Model file for the job. Use its own axes, mm. A direction names the side the tool comes from. Round coordinates to 2 decimals unless told otherwise and drop trailing zeros. Loops run counter-clockwise (first coordinate to the right, second up) from the corner with the lowest first, then second, coordinate; pieces in that order, holes last. Notation, with made-up numbers: M -19,61 L 24,61 A26 cw 24,98 Z; hole C 39.25,55 d6. An arc over 180 degrees is marked long. Use a Markdown table: item, result. Add a question column.
Item 1: Saw through at C-C on y = -239. Write the cut outline in (x, z).
Item 2: Tool access for faces 1 (the flat face through (-122, -197, 14.158)), 2 (the flat face through (-100, -220, -75.842)), 3 (the flat face through (-151.12, -291.64, 66.76)): list every direction of +Z, -Z, +X, -X, +Y, -Y with a clear straight run to the whole face (end or side of a thin tool).
Item 3: Saw through at B-B on x = -86.5. Write the cut outline in (y, z).
Item 4: Pin check, flat tips, straight feed: P1, Ø9.5, axis at x = 13, y = -14.5, coming from the +Z side; P2, Ø15.5, axis at x = -306, y = -333.5, coming from the -Z side; P3, Ø10, axis at x = -260.5, z = 41.5, coming from the -Y side; P4, Ø10, axis at y = -299.5, z = -12.5, coming from the +X side. Stop position of each tip, or through.
Item 5: Wall check: L1, parallel to Z at x = -208, y = -295; L2, parallel to Z at x = -193.5, y = -272; L3, parallel to X at y = -329, z = -60. Give the ranges that are in metal, low to high. Write a range as from..to.
Item 6: Two-plate mould, pull along Y, no slides. Class faces 4 (the flat face through (-27.86, -168.38, 66.76)), 5 (the cylindrical face through (34.67, -15.25, -43.1)), 6 (the flat face through (-304, -337, 59.158)), 7 (the flat face through (-264.9, -309.65, 0)): +Y half, -Y half, draft (parallel to the pull), parting line (faces both ways), or undercut.
Item 7: Saw through at D-D on z = 29. Write the cut outline in (x, y).
Item 8: Saw through at A-A on z = 6.5. Write the cut outline in (x, y), then the cut area to 3 significant figures.
```python
from build123d import *

# Parameters (mm, degrees)
F1_ANGLE       = 90
F2_W           = 35
F2_H           = 35
F2_R           = 7.5
F3_ANGLE       = 5
F4_ANGLE_START = 270
F4_ANGLE       = 5
F5_W           = 10
F5_H           = 120
F6_ANGLE_START = 280
F6_ANGLE       = 70
F7_W           = 35
F7_H           = 15
F8_ANGLE_START = 30
F8_ANGLE       = 30
F10_DEPTH      = 15


with BuildPart() as f1:
    # F0 (on Front) → F1 (revolve)
    with BuildSketch(Plane.XZ):
        Polygon((0, -75.8424619118), (0, 74.1575380882), (-42.5, 74.1575380882), (-42.5, 14.1575380882), (-32.5, 14.1575380882), (-32.5, 59.1575380882), (-10, 59.1575380882), (-10, -75.8424619118), align=None)
    revolve(axis=Axis((-319.5, 0, -5.3764432669), (0, 0, -1)), revolution_arc=F1_ANGLE)

    # F2 (on face) → F3 (revolve)
    with BuildSketch(Plane(origin=(-319.5, 0, 0), x_dir=(0, -1, 0), z_dir=(-1, 0, 0))):
        with Locations((337, 41.6575380882)):
            Rectangle(F2_W, F2_H)
        with Locations((337, 41.6575380882)):
            Circle(F2_R, mode=Mode.SUBTRACT)
        with Locations((337, -43.3424619118)):
            Rectangle(F2_W, F2_H)
        with Locations((337, -43.3424619118)):
            Circle(F2_R, mode=Mode.SUBTRACT)
    revolve(axis=Axis((-319.5, 0, 7.2890669107), (0, 0, 1)), revolution_arc=F3_ANGLE)

    # F2 (on face) → F4 (revolve)
    with BuildSketch(Plane(origin=(-319.5, 0, 0), x_dir=(0, -1, 0), z_dir=(-1, 0, 0)), mode=Mode.PRIVATE) as f4_sk:
        with Locations((337, 41.6575380882)):
            Rectangle(F2_W, F2_H)
        with Locations((337, 41.6575380882)):
            Circle(F2_R, mode=Mode.SUBTRACT)
        with Locations((337, -43.3424619118)):
            Rectangle(F2_W, F2_H)
        with Locations((337, -43.3424619118)):
            Circle(F2_R, mode=Mode.SUBTRACT)
    revolve(f4_sk.sketch.rotate(Axis((-319.5, 0, 74.1575380882), (0, 0, -1)), F4_ANGLE_START), axis=Axis((-319.5, 0, 74.1575380882), (0, 0, -1)), revolution_arc=F4_ANGLE)

    # F5 (on Front) → F6 (revolve, cut)
    with BuildSketch(Plane.XZ, mode=Mode.PRIVATE) as f6_sk:
        with Locations((-5, -0.8424619118)):
            Rectangle(F5_W, F5_H)
    revolve(f6_sk.sketch.rotate(Axis((-319.5, 0, -29.9057289958), (0, 0, 1)), F6_ANGLE_START), axis=Axis((-319.5, 0, -29.9057289958), (0, 0, 1)), revolution_arc=F6_ANGLE, mode=Mode.SUBTRACT)

    # F7 (on Front) → F8 (revolve)
    with BuildSketch(Plane.XZ, mode=Mode.PRIVATE) as f8_sk:
        with Locations((17.5, 66.6575380882)):
            Rectangle(F7_W, F7_H)
    revolve(f8_sk.sketch.rotate(Axis((-319.5, 0, -44.4073081017), (0, 0, -1)), F8_ANGLE_START), axis=Axis((-319.5, 0, -44.4073081017), (0, 0, -1)), revolution_arc=F8_ANGLE)

    # F9 (on face) → F10 (cut)
    with BuildSketch(Plane.XY.offset(74.1575380882)):
        with BuildLine():
            ThreePointArc((-128.7858349133, -272.3680547261), (-123.9019759301, -268.8822474243), (-119.0818139536, -265.3088779176))
            ThreePointArc((-119.0818139536, -265.3088779176), (-126.8087717489, -260.5320409865), (-135.6687521495, -262.5382301946))
            Line((-135.6687521495, -262.5382301946), (-128.7858349133, -272.3680547261))
        make_face()
        with BuildLine():
            ThreePointArc((-138.7382619085, -279.07247095), (-125.2807759939, -283.8447512008), (-116.7858349133, -272.3680547261))
            ThreePointArc((-116.7858349133, -272.3680547261), (-117.3742563302, -268.6564682402), (-119.0818139536, -265.3088779176))
            ThreePointArc((-119.0818139536, -265.3088779176), (-123.9019759301, -268.8822474243), (-128.7858349133, -272.3680547261))
            ThreePointArc((-128.7858349133, -272.3680547261), (-133.7318004616, -275.7651646606), (-138.7382619085, -279.07247095))
        make_face()
        with BuildLine():
            ThreePointArc((-135.6687521495, -262.5382301946), (-140.5842451107, -270.1777312768), (-138.7382619085, -279.07247095))
            ThreePointArc((-138.7382619085, -279.07247095), (-133.7318004616, -275.7651646606), (-128.7858349133, -272.3680547261))
            Line((-128.7858349133, -272.3680547261), (-135.6687521495, -262.5382301946))
        make_face()
        with BuildLine():
            ThreePointArc((-92.8722766297, -226.6277233703), (-96.3865067666, -235.0047296602), (-93.0240128621, -243.4437866324))
            ThreePointArc((-93.0240128621, -243.4437866324), (-88.6679185241, -239.3173628501), (-84.3869952555, -235.1130047445))
            Line((-84.3869952555, -235.1130047445), (-92.8722766297, -226.6277233703))
        make_face()
        with BuildLine():
            ThreePointArc((-84.3869952555, -235.1130047445), (-88.6679185241, -239.3173628501), (-93.0240128621, -243.4437866324))
            ThreePointArc((-93.0240128621, -243.4437866324), (-79.8950141379, -246.2405429107), (-72.3869952555, -235.1130047445))
            ThreePointArc((-72.3869952555, -235.1130047445), (-73.3423272511, -230.4209573585), (-76.0562133676, -226.4759871379))
            ThreePointArc((-76.0562133676, -226.4759871379), (-80.1826371499, -230.8320814759), (-84.3869952555, -235.1130047445))
        make_face()
        with BuildLine():
            ThreePointArc((-76.0562133676, -226.4759871379), (-84.4952703398, -223.1134932334), (-92.8722766297, -226.6277233703))
            Line((-92.8722766297, -226.6277233703), (-84.3869952555, -235.1130047445))
            ThreePointArc((-84.3869952555, -235.1130047445), (-80.1826371499, -230.8320814759), (-76.0562133676, -226.4759871379))
        make_face()
        with BuildLine():
            ThreePointArc((-47.1319452739, -190.7141650867), (-51.2073455895, -196.4059611859), (-55.4016699554, -202.010697904))
            ThreePointArc((-55.4016699554, -202.010697904), (-40.7985475105, -203.1996796044), (-33.1319452739, -190.7141650867))
            ThreePointArc((-33.1319452739, -190.7141650867), (-34.7825326257, -184.1193180647), (-39.3450891659, -179.0795240543))
            ThreePointArc((-39.3450891659, -179.0795240543), (-43.1772754806, -184.9378325658), (-47.1319452739, -190.7141650867))
        make_face()
        with BuildLine():
            ThreePointArc((-58.600073894, -182.6840949778), (-60.9440815462, -192.9999672643), (-55.4016699554, -202.010697904))
            ThreePointArc((-55.4016699554, -202.010697904), (-51.2073455895, -196.4059611859), (-47.1319452739, -190.7141650867))
            Line((-47.1319452739, -190.7141650867), (-58.600073894, -182.6840949778))
        make_face()
        with BuildLine():
            ThreePointArc((-47.1319452739, -190.7141650867), (-43.1772754806, -184.9378325658), (-39.3450891659, -179.0795240543))
            ThreePointArc((-39.3450891659, -179.0795240543), (-49.7080226626, -176.953212166), (-58.600073894, -182.6840949778))
            Line((-58.600073894, -182.6840949778), (-47.1319452739, -190.7141650867))
        make_face()
    extrude(amount=-F10_DEPTH, mode=Mode.SUBTRACT)


solid = f1.part
```
Entries:
| question | item | result |
|---|---|---|
| 1 | outline | M -179.47,14.16 L -160.6,14.16 L -160.6,59.16 L -95.74,59.16 L -95.74,74.16 L -179.47,74.16 Z; M -122.86,-75.84 L -107.46,-75.84 L -107.46,-60.84 L -122.86,-60.84 Z; M -73.03,59.16 L -57.68,59.16 L -57.68,74.16 L -73.03,74.16 Z |
| 2 | face 1 | -Z, -X, +Y |
| 2 | face 2 | -Z, +X, -X, +Y, -Y |
| 2 | face 3 | +Z, -Z, -Y |
| 3 | outline | M -267.17,59.16 L -246.93,59.16 L -246.93,74.16 L -267.17,74.16 Z; M -223.3,59.16 L -167.57,59.16 L -167.57,14.16 L -149.8,14.16 L -149.8,74.16 L -223.3,74.16 Z; M -218.61,-75.84 L -203.72,-75.84 L -203.72,-60.84 L -218.61,-60.84 Z |
| 4 | P1 | z = 59.16 |
| 4 | P2 | z = -60.84 |
| 4 | P3 | y = -314.9 |
| 4 | P4 | through |
| 5 | L1 | -75.84..-60.84, 59.16..74.16 |
| 5 | L2 | 59.16..74.16 |
| 5 | L3 | -319.5..-290.72 |
| 6 | face 4 | undercut |
| 6 | face 5 | -Y half |
| 6 | face 6 | draft |
| 6 | face 7 | undercut |
| 7 | outline | M -319.5,-354.5 A354.5 ccw -288.6,-353.15 L -291.65,-318.28 A319.5 ccw -264.02,-314.65 L -265.76,-304.8 A309.5 cw -319.5,-309.5 Z; M -319.5,-287 A287 ccw -32.5,0 L -42.5,0 A277 cw -319.5,-277 Z; M -14.7,-53.74 L -4.85,-55.48 A319.5 ccw -1.22,-27.85 L 33.65,-30.9 A354.5 ccw 35,0 L -10,0 A309.5 cw Z |
| 8 | outline | M -319.5,-319.5 A319.5 ccw -264.02,-314.65 L -265.76,-304.8 A309.5 cw -319.5,-309.5 Z; M -14.7,-53.74 L -4.85,-55.48 A319.5 ccw 0,0 L -10,0 A309.5 cw Z |
| 8 | area | 1,100 mm2 |
